Geometry: see drawing. Coordinates: mm, zero at the bounding-box minimum. A direction names the side the tool comes from. Give positions to 0.01 mm unless a question says otherwise; leave off trailing zeros. Write each loop counter-clockwise with the first axis right and the second up, starting at its lowest first coordinate (ties: lowest second). Pieces come first, ordered by that corner, then holes. Notation, with made-up numbers: M -29.5,51 L -20.5,51 A30 ccw -20.5,85 Z; hole C 30,0 d6. An arc over 180 degrees is marked long. Use one line per item in the form item = value. Start each with the question number.
Item 1: Section query D-D on z = 10.5. Return loops of the section in (x, y), then the cut area to 3 significant figures.
Item 2: Section query C-C on y = 12. Return loops of the section in (x, z).
Item 3: Contact query for flat-ended pins moving along their axis: P1, Ø5, axis at x = 6.5, y = 13, coming from the -Z side; P2, Ø1.5, axis at x = 4, z = 5, coming from the +Y side; P3, Ø6, axis at x = 9.5, z = 8, coming from the +Y side. Output: stop coordinate, or through.
Item 4: Section query A-A on x = 5.75. Return loops of the section in (y, z), then the cut area to 3 significant figures.
Item 5: Material intervals for line 1 along Z through (x, y) = (8.5, 8.75); line 2 along Z through (x, y) = (4, 10.75); line 3 along X through (y, z) = (18.5, 22), sorted ascending. Write a range as from..to.
Item 6: Access query for the marked faces 3 and 4. Directions: +Z, -Z, +X, -X, +Y, -Y. A direction counts if a zero-diameter tool reaches every point of the face in a straight line with its end or side. Return the directions, or none.
Item 7: Section query B-B on z = 35. Return loops of the section in (x, y).
Item 8: Pull-direction query (Z, two-part tool) for the marked faces 1 and 2; classes: released by +Z, released by -Z, zero draft, split by the parting line, or undercut.
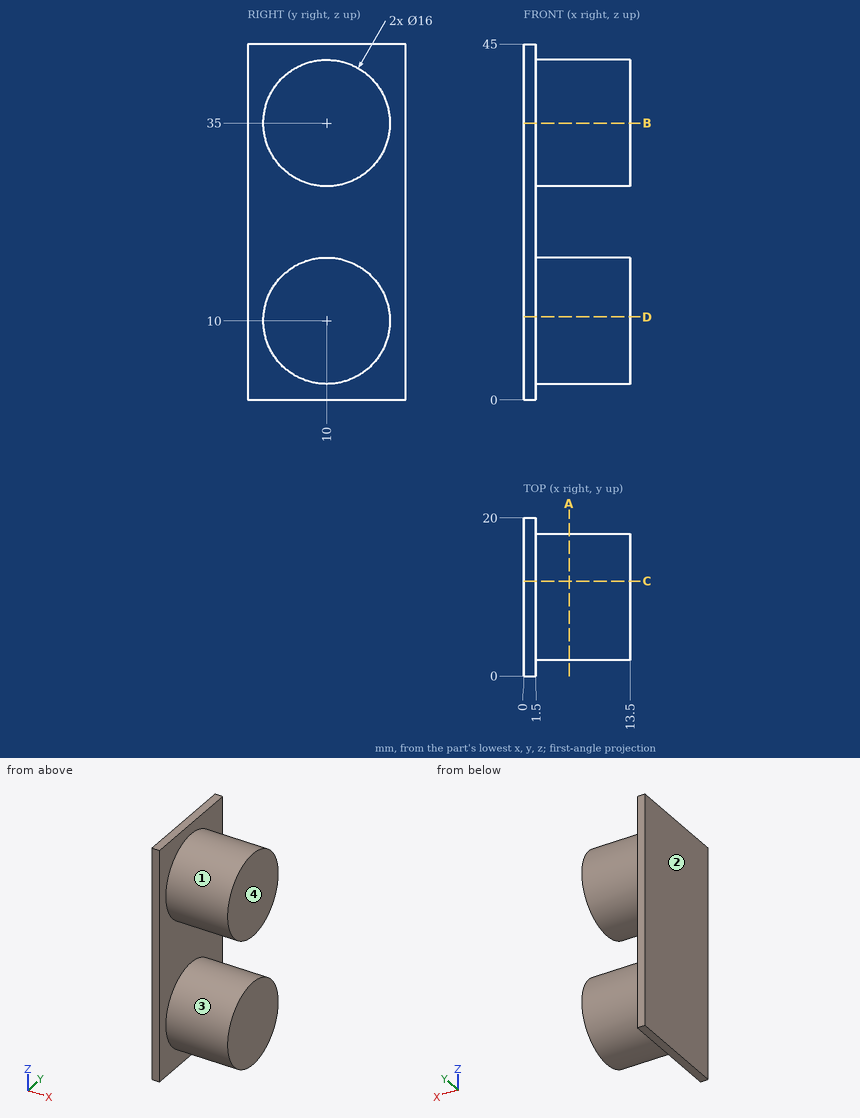
Answer sheet:
q1.outline = M 0,0 L 1.5,0 L 1.5,2.02 L 13.5,2.02 L 13.5,17.98 L 1.5,17.98 L 1.5,20 L 0,20 Z
q1.area = 222 mm2
q2.outline = M 0,0 L 1.5,0 L 1.5,2.25 L 13.5,2.25 L 13.5,17.75 L 1.5,17.75 L 1.5,27.25 L 13.5,27.25 L 13.5,42.75 L 1.5,42.75 L 1.5,45 L 0,45 Z
q3.P1 = 2.02
q3.P2 = 16.78
q3.P3 = 18
q4.outline = C 10,10 d16; C 10,35 d16
q4.area = 402 mm2
q5.line_1 = 2.1..17.9, 27.1..42.9
q5.line_2 = 2.04..17.96, 27.04..42.96
q5.line_3 = 0..1.5
q6.face_3 = +X
q6.face_4 = +Z, -Z, +X, +Y, -Y
q7.outline = M 0,0 L 1.5,0 L 1.5,2 L 13.5,2 L 13.5,18 L 1.5,18 L 1.5,20 L 0,20 Z
q8.face_1 = undercut
q8.face_2 = zero draft
